Input: part model. Units: mm. Frame: model coordinates. Give positions to 0.01 mm unless a question says otherwise; leave off trailing zeros. Write each loop counter-clockwise with the first axis right and the second up, starting at its lowest first coordinate (ties: lowest second). Pieces come first, ordered by that corner, then holes.
```python
from build123d import *

# Parameters (mm, degrees)
F0_R     = 10
F0_R_2   = 2.45
F1_DEPTH = 3
F2_R     = 3.75
F2_R_2   = 2.45
F3_DEPTH = 4
F4_SIZE  = 0.5


with BuildPart() as f1:
    # F0 (on Top) → F1 (new body)
    with BuildSketch(Plane.XY):
        Circle(F0_R)
        Circle(F0_R_2, mode=Mode.SUBTRACT)
    extrude(amount=F1_DEPTH)

    # F2 (on face) → F3 (join)
    with BuildSketch(Plane.XY.offset(3)):
        Circle(F2_R)
        Circle(F2_R_2, mode=Mode.SUBTRACT)
    extrude(amount=F3_DEPTH)

    # F4
    f4_edges = [f1.edges().sort_by_distance(p)[0] for p in [
        (-10, 0, 3),
        (-2.45, 0, 7),
        (-10, 0, 0),
        (-2.45, 0, 0),
    ]]
    chamfer(f4_edges, length=F4_SIZE)


solid = f1.part
```
Item 1: Ray query, line 1 (Y direction, x = 0, z = 2); line 2 (Y direction, x = 0, z = 3.85); line 3 (Z direction, x = 1.5, y = 9). Return the intervals inside material, ascending.
Item 2: Section C-C (z = 2.25). Return loops of the section in (x, y).
Item 3: Pin query (flat end, axial travel): pin 1 (1.5 mm diameter, centred on x = -6.5, z = 1, fed in from -Y); pin 2 (5.5 mm diameter, centred on x = 1.5, y = 2, fed in from +Z); pin 3 (2 mm diameter, centred on x = -1, y = 1, fed in from +Z); pin 4 (1.5 mm diameter, centred on y = -2, z = 1.5, fed in from +X). Return the tip coordinate at first contact, or that it passes through.
Item 4: Section A-A (y = 0). Return loops of the section in (x, z), and give its area (3 significant figures).
Item 5: Section D-D (z = 6.75). Return loops of the section in (x, y), and give its area (3 significant figures).
Item 6: Mould query, pull axis Y, two halves, no side actions, for faces 1 (the cylindrical face through (-3.746, 0.165, 4.972)), 2 (the flat face through (4, 0, 3)), 3 (the cylindrical face through (-0.5, -2.4, 3.5)). Classes: +Y half, -Y half, draft (parallel to the pull), parting line (faces both ways), or undercut.
Solved:
1. line 1: y = -10 to -2.45, 2.45 to 10
1. line 2: y = -3.75 to -2.45, 2.45 to 3.75
1. line 3: z = 0 to 3
2. outline: circle Ø20 at (0, 0); hole circle Ø4.9 at (0, 0)
3. pin 1: stops at y = -8.18
3. pin 2: stops at z = 7
3. pin 3: passes through
3. pin 4: stops at x = 9.92
4. outline: (-10, 0.5) - (-9.5, 0) - (-2.95, 0) - (-2.45, 0.5) - (-2.45, 6.5) - (-2.95, 7) - (-3.75, 7) - (-3.75, 3) - (-9.5, 3) - (-10, 2.5) - close; (2.45, 0.5) - (2.95, 0) - (9.5, 0) - (10, 0.5) - (10, 2.5) - (9.5, 3) - (3.75, 3) - (3.75, 7) - (2.95, 7) - (2.45, 6.5) - close
4. area: 54.7 mm2
5. outline: circle Ø7.5 at (0, 0); hole circle Ø5.4 at (0, 0)
5. area: 21.3 mm2
6. face 1: parting line
6. face 2: draft
6. face 3: undercut
